from build123d import *

# Parameters (mm, degrees)
F0_W     = 13.333333
F0_H     = 5.842
F0_W_2   = 5.842
F0_H_2   = 5
F0_H_3   = 20
F1_DEPTH = 5.842


with BuildPart() as f1:
    # F0 (on Front) → F1 (new body)
    with BuildSketch(Plane.XZ):
        Polygon((-20, 60), (-25, 60), (-25, 55), (-25, 50), (-25, 30), (-25, 10), (-25, -10), (-25, -30), (-25, -50), (-25, -55), (-25, -60), (-20, -60), (-6.666667, -60), (6.666667, -60), (20, -60), (25, -60), (25, -55), (25, -50), (25, -30), (25, -10), (25, 10), (25, 30), (25, 50), (25, 55), (25, 60), (20, 60), (6.666667, 60), (-6.666667, 60), align=None)
        with Locations((-13.333334, 62.921)):
            Rectangle(F0_W, F0_H)
        with Locations((-27.921, 52.5)):
            Rectangle(F0_W_2, F0_H_2)
        with Locations((13.333334, 62.921)):
            Rectangle(F0_W, F0_H)
        with Locations((-27.921, 20)):
            Rectangle(F0_W_2, F0_H_3)
        with Locations((-27.921, -20)):
            Rectangle(F0_W_2, F0_H_3)
        with Locations((27.921, 52.5)):
            Rectangle(F0_W_2, F0_H_2)
        with Locations((-27.921, -52.5)):
            Rectangle(F0_W_2, F0_H_2)
        with Locations((27.921, 20)):
            Rectangle(F0_W_2, F0_H_3)
        with Locations((27.921, -20)):
            Rectangle(F0_W_2, F0_H_3)
        with Locations((-13.333334, -62.921)):
            Rectangle(F0_W, F0_H)
        with Locations((27.921, -52.5)):
            Rectangle(F0_W_2, F0_H_2)
        with Locations((13.333334, -62.921)):
            Rectangle(F0_W, F0_H)
    extrude(amount=F1_DEPTH)


solid = f1.part
CAD build for the part. Positions are in the model's coordinates, mm. A direction names the side the tool comes from. Round coordinates to 2 decimals unless told otherwise and drop trailing zeros. Write each loop counter-clockwise with the first axis right and the second up, starting at its lowest first coordinate (ties: lowest second). Pieces come first, ordered by that corner, then holes. Notation, with made-up numbers: M 9.25,85 L 50.25,85 A38 ccw 50.25,123 Z; hole C -24,-13 d9. An arc over 180 degrees is marked long. Use a Markdown table: item, result. Add a question column.
1. Slice it at A-A on x = 22.5. Give the cut face in (y, z), then the cut area to 3 significant figures.
2. Pull direction Z, two halves, no side cores. Call faces 1 (the face through (30.842, -3, 20)), 2 (the face through (0, -3, 60)), 3 (the face through (28, -3, 50)): released by +Z, released by -Z, zero draft, split by the parting line, or undercut.
3. Drill centre lines: probe 1 along Z at (x, y) = (28.5, -1.55); probe 2 along Z at (x, y) = (-2, -3.3); probe 3 along X at (y, z) = (-4.3, -58). Where is each one in solid material? Low to high.
4. Slice it at B-B on z = 3. Give the cut face in (x, y), then the cut area to 3 significant figures.
5. 3-axis set-ups, long thin cutter, end or side, ignore diameter. For faces 4 (the face through (-28, -3, -50)), 5 (the face through (-28, -3, -55)), 6 (the face through (6.667, -3, 63)), 7 (the face through (28, -3, -10)): which of +Z, -Z, +X, -X, +Y, -Y reach the whole face in a straight line?
6. Flat gauge pins, fed straight in: P1, Ø1.8, axis at x = -27, y = -4, coming from the -Z side; P2, Ø1.5, axis at x = -2, y = -2.5, coming from the -Z side; P3, Ø2, axis at x = 14, z = -13, coming from the +Y side; P4, Ø3, axis at x = 28, y = -4, coming from the +Z side. Where does each tip first touch, or does it go through?
Reply:
| question | item | result |
|---|---|---|
| 1 | outline | M -5.84,-60 L 0,-60 L 0,60 L -5.84,60 Z |
| 1 | area | 701 mm^2 |
| 2 | face 1 | zero draft |
| 2 | face 2 | released by +Z |
| 2 | face 3 | undercut |
| 3 | probe 1 | z = -55 to -50, -30 to -10, 10 to 30, 50 to 55 |
| 3 | probe 2 | z = -60 to 60 |
| 3 | probe 3 | x = -25 to 25 |
| 4 | outline | M -25,-5.84 L 25,-5.84 L 25,0 L -25,0 Z |
| 4 | area | 292 mm^2 |
| 5 | face 4 | -X, +Y, -Y |
| 5 | face 5 | -Z, -X, +Y, -Y |
| 5 | face 6 | +Z, +Y, -Y |
| 5 | face 7 | +X, +Y, -Y |
| 6 | P1 | stops at z = -55 |
| 6 | P2 | stops at z = -60 |
| 6 | P3 | stops at y = 0 |
| 6 | P4 | stops at z = 55 |
